```python
from build123d import *

# Parameters (mm, degrees)
F1_DEPTH = 1
F2_W     = 2.5
F2_H     = 5
F3_DEPTH = 2.5
F5_DEPTH = 0.1


# Not quite as in the source:
# - a feature names something its author has since deleted; it is built from what else it names


with BuildPart() as f1:
    # F0 (on Top) → F1 (new body)
    with BuildSketch(Plane.XY):
        with BuildLine():
            Line((0, 3.5), (-13.5, 3.5))
            ThreePointArc((-13.5, 3.5), (-17, 0), (-13.5, -3.5))
            Line((-13.5, -3.5), (0, -3.5))
            Line((0, -3.5), (13.5, -3.5))
            ThreePointArc((13.5, -3.5), (17, 0), (13.5, 3.5))
            Line((13.5, 3.5), (0, 3.5))
        make_face()
    extrude(amount=F1_DEPTH)

    # F2 (on face) → F3 (join)
    with BuildSketch(Plane.XY.offset(1)):
        with Locations((-12.25, 0)):
            Rectangle(F2_W, F2_H)
        with Locations((12.25, 0)):
            Rectangle(F2_W, F2_H)
        with Locations((-8.75, 0)):
            Rectangle(F2_W, F2_H)
        with Locations((-5.25, 0)):
            Rectangle(F2_W, F2_H)
        with Locations((-1.75, 0)):
            Rectangle(F2_W, F2_H)
        with Locations((1.75, 0)):
            Rectangle(F2_W, F2_H)
        with Locations((5.25, 0)):
            Rectangle(F2_W, F2_H)
        with Locations((8.75, 0)):
            Rectangle(F2_W, F2_H)
    extrude(amount=F3_DEPTH)

    # F4 (on face) → F5 (cut)
    with BuildSketch(Plane.XY.offset(1)):
        with BuildLine():
            ThreePointArc((-15.75, 0), (-15.25, -0.5), (-14.75, 0))
            ThreePointArc((-14.75, 0), (-15.25, 0.5), (-15.75, 0))
        make_face()
    extrude(amount=-F5_DEPTH, mode=Mode.SUBTRACT)


solid = f1.part
```
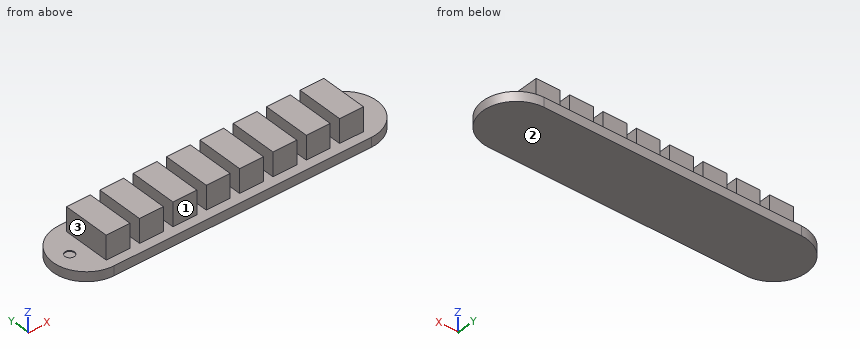
Check sheet for the modelled part. Datum: model origin and axes. Units: mm. Face numbers are marked on the shaded views. A direction names the side the tool comes from. Round coordinates to 2 decimals unless told otherwise and drop trailing zeros. Loops run counter-clockwise (first coordinate to the right, second up) from the corner with the lowest first, then second, coordinate; pieces in that order, holes last. Notation, with made-up numbers: (7.25, 38) -> (13.25, 38) arc R11 cw to (13.25, 53) -> close; hole circle Ø10 at (55.5, 46). An arc over 180 degrees is marked (long way). Answer in a Markdown table with one row per item.
Q1. Sectioned sample at A-A on x = -2. Enter the section's corners in (y, z), then the cut area to 3 significant figures.
Data:
| item | result |
|---|---|
| outline | (-3.5, 0) -> (3.5, 0) -> (3.5, 1) -> (2.5, 1) -> (2.5, 3.5) -> (-2.5, 3.5) -> (-2.5, 1) -> (-3.5, 1) -> close |
| area | 19.5 mm^2 |
Q2. Sectioned sample at B-B on x = -15.25. Enter the section's corners in (y, z), then the cut area to 3 significant figures.
Data:
| item | result |
|---|---|
| outline | (-3.03, 0) -> (3.03, 0) -> (3.03, 1) -> (0.5, 1) -> (0.5, 0.9) -> (-0.5, 0.9) -> (-0.5, 1) -> (-3.03, 1) -> close |
| area | 5.96 mm^2 |
Q3. Sectioned sample at C-C on x = 15.5. Enter the section's corners in (y, z), then the cut area to 3 significant figures.
Data:
| item | result |
|---|---|
| outline | (-2.87, 0) -> (2.87, 0) -> (2.87, 1) -> (-2.87, 1) -> close |
| area | 5.74 mm^2 |
Q4. Go/stop test with flat-tipped pins: P1, Ø0.8, axis at x = -15.5, y = 0, coming from the +Z side; P2, Ø2, axis at y = 2.5, z = 1, coming from the +X side; P3, Ø0.8, axis at x = -5.5, z = 2, coming from the +Y side. Record where each tip stops, or that it passes through.
Data:
| item | result |
|---|---|
| P1 | stops at z = 1 |
| P2 | stops at x = 16.66 |
| P3 | stops at y = 2.5 |
Q5. Set-up check for the marked faces 1, 2 and 3: record each of +Z, -Z, +X, -X, +Y, -Y from which the full face is reachable in a straight line by a thin tool's end or side.
Data:
| item | result |
|---|---|
| face 1 | +Z, +X, -X, -Y |
| face 2 | -Z, +X, -X, +Y, -Y |
| face 3 | +Z, -X, +Y, -Y |
Q6. Thickness scan on L1, parallel to Y at x = 2, z = 2.6; L2, parallel to Z at x = 1.5, y = 2.75; L3, parallel to X at y = -2.5, z = 0.55. Record the ranges inside material, lowest first.
Data:
| item | result |
|---|---|
| L1 | y = -2.5 to 2.5 |
| L2 | z = 0 to 1 |
| L3 | x = -15.95 to 15.95 |
